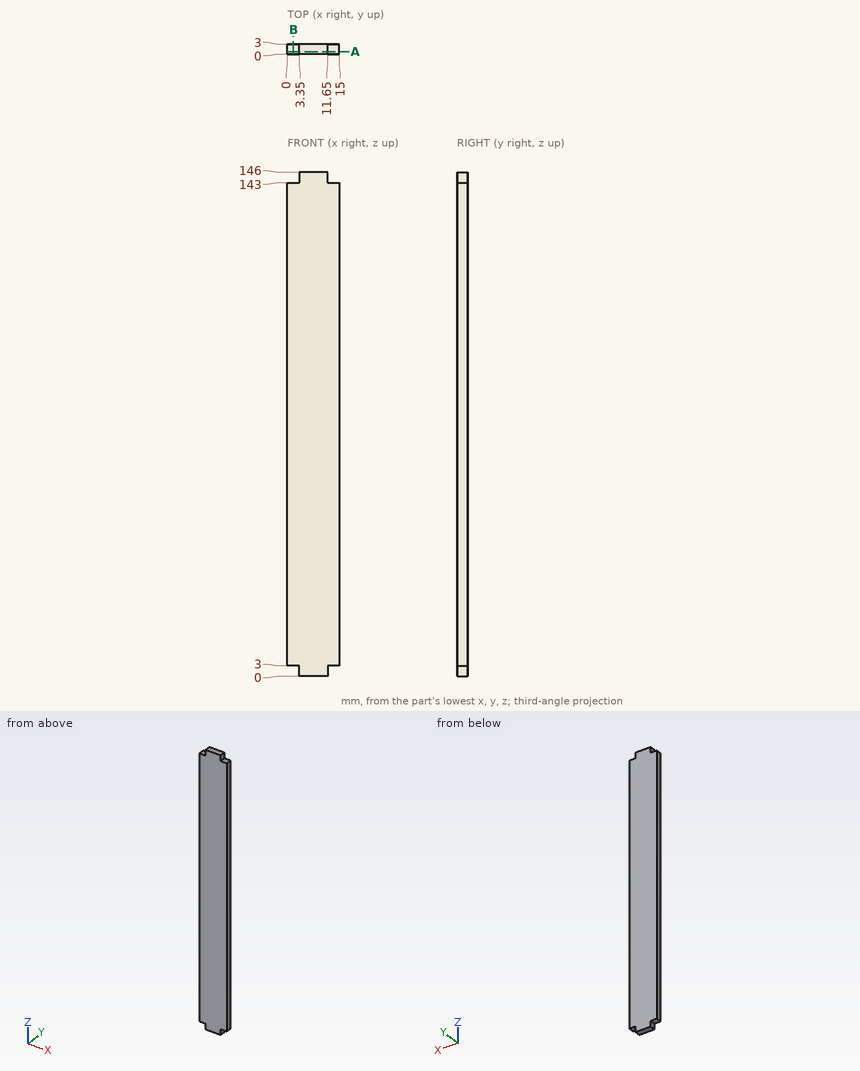
Design review of the part shown in the three views and the two pictorial views. Dimensions are in mm from the part's minimum x, y and z. Coordinates: 2 decimals unless noted, no trailing zeros. Loops run counter-clockwise (first coordinate to the right, second up) from the corner with the lowest first, then second, coordinate; pieces in that order, holes last. Notation, with made-up numbers: (65.5, 82) -> (77.5, 82) arc R33 ccw to (77.5, 117) -> close; hole circle Ø4 at (58.25, -18.5). An arc over 180 degrees is marked (long way). Answer as CSV lines item,"result".
Item 1: Take a section at A-A, the plane y = 0.8. State the section outline as (x, z) points, and give its area (3 significant figures).
Results below:
outline,"(0, 3) -> (3.35, 3) -> (3.35, 0) -> (11.65, 0) -> (11.65, 3) -> (15, 3) -> (15, 143) -> (11.65, 143) -> (11.65, 146) -> (3.35, 146) -> (3.35, 143) -> (0, 143) -> close"
area,"2,150 mm2"
Item 2: For L1, parallel to Z at x = 13.5, y = 0.45, list the stretches that pass through material, from the lowest coordinate up.
Results below:
L1,"z = 3 to 143"
Item 3: Take a section at B-B, the plane x = 1.75. State the section outline as (y, z) points, and give its area (3 significant figures).
Results below:
outline,"(0, 3) -> (3, 3) -> (3, 143) -> (0, 143) -> close"
area,"420 mm2"
Item 4: Insertion check: pin 1 (0.9 mm diameter, centred on y = 1, z = 1, fed in from +X); pin 2 (1.5 mm diameter, centred on x = 12.5, y = 1, fed in from -Z); pin 3 (0.9 mm diameter, centred on x = 13.5, y = 2, fed in from +Z). Each pin has a flat end and moves straight along its axis. Give the tip position at first contact, or say it passes through.
Results below:
pin 1,"stops at x = 11.65"
pin 2,"stops at z = 3"
pin 3,"stops at z = 143"
